from build123d import *

# Parameters (mm, degrees)
F0_R     = 4
F1_DEPTH = 3
F2_R     = 6
F3_DEPTH = 10
F4_R     = 2.5
F5_DEPTH = 2
F6_R     = 1.5
F7_R     = 2.5
F8_DEPTH = 8


with BuildPart() as f1:
    # F0 (on Top) → F1 (new body)
    with BuildSketch(Plane.XY):
        Circle(F0_R)
    extrude(amount=F1_DEPTH)

    # F2 (on face) → F3 (join)
    with BuildSketch(Plane.XY.offset(3)):
        Circle(F2_R)
    extrude(amount=F3_DEPTH)

    # F4 (on face) → F5 (join)
    with BuildSketch(Plane.XY.offset(13)):
        Circle(F4_R)
    extrude(amount=F5_DEPTH)

    # F6
    f6_edges = [f1.edges().sort_by_distance(p)[0] for p in [
        (-6, 0, 13),
        (-6, 0, 3),
    ]]
    fillet(f6_edges, radius=F6_R)

    # F7 (on face) → F8 (cut)
    with BuildSketch(Plane(origin=(0, 0, 0), x_dir=(1, 0, 0), z_dir=(0, 0, -1))):
        Circle(F7_R)
    extrude(amount=-F8_DEPTH, mode=Mode.SUBTRACT)


solid = f1.part
The listing builds one solid part. Answer for the finished solid, in the listing's coordinates (mm). A direction names the side the tool comes from. Coordinates: 2 decimals unless noted, no trailing zeros. Write each loop counter-clockwise with the first axis right and the second up, starting at its lowest first coordinate (ties: lowest second). Pieces come first, ordered by that corner, then holes. Notation, with made-up numbers: (-15.75, 13) - (38.25, 13) arc R11 ccw to (38.25, 17) - close; hole circle Ø6 at (44.5, 51.5). An arc over 180 degrees is marked (long way). Return JSON: item names as keys, results as strings.
1. The part is cut by section A-A on y = 0. Determine the outline of the cut face in (x, z).
Final values:
{"outline": "(-6, 4.5) arc R1.5 ccw to (-4.5, 3) - (-4, 3) - (-4, 0) - (-2.5, 0) - (-2.5, 8) - (2.5, 8) - (2.5, 0) - (4, 0) - (4, 3) - (4.5, 3) arc R1.5 ccw to (6, 4.5) - (6, 11.5) arc R1.5 ccw to (4.5, 13) - (2.5, 13) - (2.5, 15) - (-2.5, 15) - (-2.5, 13) - (-4.5, 13) arc R1.5 ccw to (-6, 11.5) - close"}
2. The part is cut by section C-C on z = 8.75. Determine the outline of the cut face in (x, y), then the cut area to 3 significant figures.
Final values:
{"outline": "circle Ø12 at (0, 0)", "area": "113 mm^2"}
3. Which of the six approach directions +Z, -Z, +X, -X, +Y, -Y give full straight-line access (tool end or side, diameter ignored) to faces 1 (the face through (0, 0, 15)), 2 (the face through (2, -2, 13)), 3 (the face through (0, 0, 8))?
Final values:
{"face 1": "+Z, +X, -X, +Y, -Y", "face 2": "+Z", "face 3": "-Z"}
4. Consider line 1 along Y through (x, z) = (0, 2); line 2 along Z through (x, y) = (1.75, 2); line 3 along Y through (x, z) = (0, 4.5). Determine where each line is inside the solid, lowest interval first.
Final values:
{"line 1": "-4 to -2.5, 2.5 to 4", "line 2": "0 to 13", "line 3": "-6 to -2.5, 2.5 to 6"}
5. Each of these flat-tipped pins is pushed along its axis until it touches: pin 1 Ø3 at (x, z) = (-3, 10) entering from +Y; pin 2 Ø6 at (y, z) = (4.5, 2.5) entering from +X; pin 3 Ø1 at (y, z) = (-1.5, 11.5) entering from -X. Where does it stop, or does it pass through?
Final values:
{"pin 1": "y = 5.81", "pin 2": "x = 5.62", "pin 3": "x = -5.92"}
6. For a pull along X with two mould halves and no side action, classify faces 4 (the face through (-0.54, -2.44, 13.99)), 5 (the face through (-0.54, 2.44, 3.94)), 6 (the face through (-3, -3, 3)) as +X half, -X half, draft (parallel to the pull), parting line (faces both ways), or undercut.
Final values:
{"face 4": "parting line", "face 5": "undercut", "face 6": "draft"}
